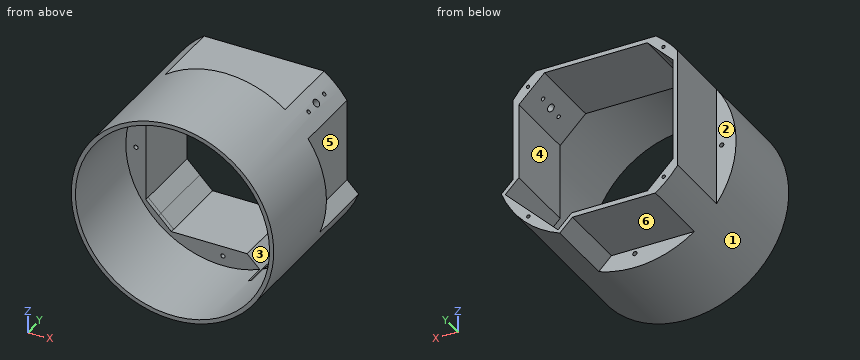
```python
from build123d import *

# Parameters (mm, degrees)
CROQUIS1_R              = 120
CROQUIS1_R_2            = 115
SALIENTE_EXTRUIR1_DEPTH = 110
CROQUIS2_R              = 120
CROQUIS2_W              = 152.253442708
CROQUIS2_H              = 152.577386202
SALIENTE_EXTRUIR2_DEPTH = 90
CORTAR_EXTRUIR1_START   = -85
CORTAR_EXTRUIR1_DEPTH   = 85
CORTAR_EXTRUIR2_DEPTH   = 30
CROQUIS5_R              = 2
CORTAR_EXTRUIR3_DEPTH   = 10
CROQUIS7_R              = 4.5
CORTAR_EXTRUIR4_DEPTH   = 343.045214483
CROQUIS8_R              = 2.25
CORTAR_EXTRUIR5_DEPTH   = 30
CROQUIS12_R             = 2.5
CORTAR_EXTRUIR7_DEPTH   = 15


with BuildPart() as part:
    # Croquis1 → Saliente-Extruir1 (new body)
    with BuildSketch(Plane(origin=(0, 0, 0), x_dir=(1, 0, 0), z_dir=(0, 1, 0))):
        with Locations(Location((0, 0, 0), (0, 0, 270))):
            Circle(CROQUIS1_R)
        with Locations(Location((0, 0, 0), (0, 0, 270))):
            Circle(CROQUIS1_R_2, mode=Mode.SUBTRACT)
    extrude(amount=SALIENTE_EXTRUIR1_DEPTH)

    # Croquis2 → Saliente-Extruir2 (add)
    with BuildSketch(Plane(origin=(0, 110, 0), x_dir=(1, 0, 0), z_dir=(0, 1, 0))):
        with Locations(Location((0, 0, 0), (0, 0, 270))):
            Circle(CROQUIS2_R)
        Rectangle(CROQUIS2_W, CROQUIS2_H, mode=Mode.SUBTRACT)
    extrude(amount=SALIENTE_EXTRUIR2_DEPTH)

    # Croquis3 → Cortar-Extruir1 (cut)
    with BuildSketch(Plane(origin=(0, 200, 0), x_dir=(1, 0, 0), z_dir=(0, 1, 0)).offset(CORTAR_EXTRUIR1_START)):
        Polygon((-45.841188947, 76.288693101), (43.949902098, 76.288693101), (28.807150506, 91.431444693), (-61.004991492, 91.431444693), align=None)
        Polygon((-91.267423391, -61.169009949), (-76.126721354, -46.007259807), (-76.126721354, 45.961058747), (-91.267423391, 61.101790004), align=None)
        Polygon((-61.028027907, -91.408376254), (61.007038201, -91.408376254), (45.887355048, -76.288693101), (-45.887325869, -76.288693101), align=None)
        Polygon((76.126721354, -46.007289027), (91.267423391, -61.147991064), (91.267423391, 28.971171808), (76.126721354, 44.111873845), align=None)
        with BuildLine():
            Line((98.300064852, 29.330876538), (98.300064852, -68.82657372))
            ThreePointArc((98.300064852, -68.82657372), (114.446511048, -36.083183186), (120, 0))
            ThreePointArc((120, 0), (119.08657738, 14.777925699), (116.360215201, 29.330876538))
            Line((116.360215201, 29.330876538), (98.300064852, 29.330876538))
        make_face()
        with BuildLine():
            Line((71.118639022, -96.654742169), (-71.118639022, -96.654742169))
            ThreePointArc((-71.118639022, -96.654742169), (0, -120), (71.118639022, -96.654742169))
        make_face()
        with BuildLine():
            Line((-96.908612184, -70.772317219), (-96.908612184, 70.772317219))
            ThreePointArc((-96.908612184, 70.772317219), (-120, 0), (-96.908612184, -70.772317219))
        make_face()
        with BuildLine():
            ThreePointArc((27.732572497, 116.751464328), (-23.555261835, 117.665413949), (-70.538900009, 97.078646393))
            Line((-70.538900009, 97.078646393), (27.732572497, 97.078646393))
            Line((27.732572497, 97.078646393), (27.732572497, 116.751464328))
        make_face()
        Polygon((76.126721354, 44.111873845), (91.267423391, 28.971171808), (107.376851904, 45.080600321), (91.267423391, 61.190028833), (61.007038201, 91.408376254), (44.895560134, 107.519854321), (28.807150506, 91.431444693), (43.949902098, 76.288693101), (76.126721354, 76.288693101), align=None)
        Polygon((61.007038201, -91.408376254), (76.126721354, -76.288693101), (45.887355048, -76.288693101), align=None)
        Polygon((76.126721354, -46.007289027), (76.126721354, -76.288693101), (91.267423391, -61.147991064), align=None)
        Polygon((-91.267423391, -61.169009949), (-76.126721354, -76.288693101), (-76.126721354, -46.007259807), align=None)
        Polygon((-76.126721354, -76.288693101), (-61.028027907, -91.408376254), (-45.887325869, -76.288693101), align=None)
        Polygon((-91.267423391, 61.101790004), (-76.126721354, 45.961058747), (-76.126721354, 76.288693101), align=None)
        Polygon((-76.126721354, 76.288693101), (-45.841188947, 76.288693101), (-61.004991492, 91.431444693), align=None)
        with BuildLine():
            Line((27.732572497, 116.751464328), (27.732572497, 97.078646393))
            Line((27.732572497, 97.078646393), (42.772301896, 112.118375793))
            ThreePointArc((42.772301896, 112.118375793), (35.32846877, 114.68173043), (27.732572497, 116.751464328))
        make_face()
        with BuildLine():
            ThreePointArc((116.360215201, 29.330876538), (114.392817368, 36.253045866), (112.014025768, 43.044837453))
            Line((112.014025768, 43.044837453), (98.300064852, 29.330876538))
            Line((98.300064852, 29.330876538), (116.360215201, 29.330876538))
        make_face()
    extrude(amount=CORTAR_EXTRUIR1_DEPTH, mode=Mode.SUBTRACT)

    # Croquis4 → Cortar-Extruir2 (cut)
    with BuildSketch(Plane(origin=(0, 115, 0), x_dir=(1, 0, 0), z_dir=(0, 1, 0))):
        Polygon((-91.267423391, 61.101790004), (-91.267423391, -61.169009949), (-61.028027907, -91.408376254), (61.007038201, -91.408376254), (91.267423391, -61.147991064), (91.267423391, 28.971171808), (107.376851904, 45.080600321), (44.895560134, 107.519854321), (28.807150506, 91.431444693), (-61.004991492, 91.431444693), align=None)
    extrude(amount=-CORTAR_EXTRUIR2_DEPTH, mode=Mode.SUBTRACT)

    # Croquis5 → Cortar-Extruir3 (cut)
    with BuildSketch(Plane(origin=(0, 200, 0), x_dir=(1, 0, 0), z_dir=(0, 1, 0))):
        with Locations(Location((80.009543849, 80.403081156, 0), (0, 0, 270))):
            Circle(CROQUIS5_R)
        with Locations(Location((-80.403081156, 80.009543849, 0), (0, 0, 270))):
            Circle(CROQUIS5_R)
        with Locations(Location((-80.009543849, -80.403081156, 0), (0, 0, 270))):
            Circle(CROQUIS5_R)
        with Locations(Location((80.403081156, -80.009543849, 0), (0, 0, 270))):
            Circle(CROQUIS5_R)
    extrude(amount=-CORTAR_EXTRUIR3_DEPTH, mode=Mode.SUBTRACT)

    # Croquis7 → Cortar-Extruir4 (cut, through all)
    with BuildSketch(Plane(origin=(76.207707227, 0, 76.207707227), x_dir=(-0.7071067811865415, 0, 0.7071067811865537), z_dir=(-0.7071067811865537, 0, -0.7071067811865415))):
        with Locations((0, 157.851936769)):
            Circle(CROQUIS7_R)
    extrude(amount=-CORTAR_EXTRUIR4_DEPTH, mode=Mode.SUBTRACT)

    # Croquis8 → Cortar-Extruir5 (cut)
    with BuildSketch(Plane(origin=(76.207707227, 0, 76.207707227), x_dir=(-0.7071067811865415, 0, 0.7071067811865537), z_dir=(-0.7071067811865537, 0, -0.7071067811865415))):
        with Locations((1.055799094, 176.265297527)):
            Circle(CROQUIS8_R)
        with Locations((-0.790662854, 139.817237098)):
            Circle(CROQUIS8_R)
    extrude(amount=-CORTAR_EXTRUIR5_DEPTH, mode=Mode.SUBTRACT)

    # Croquis12 → Cortar-Extruir7 (cut)
    with BuildSketch(Plane(origin=(0, 115, 0), x_dir=(1, 0, 0), z_dir=(0, 1, 0))):
        with Locations(Location((102.928666222, 0, 0), (0, 0, 270))):
            Circle(CROQUIS12_R)
        with Locations(Location((0, -102.928666222, 0), (0, 0, 270))):
            Circle(CROQUIS12_R)
        with Locations(Location((-102.928666222, 0, 0), (0, 0, 270))):
            Circle(CROQUIS12_R)
        with Locations(Location((0, 102.928666222, 0), (0, 0, 270))):
            Circle(CROQUIS12_R)
    extrude(amount=-CORTAR_EXTRUIR7_DEPTH, mode=Mode.SUBTRACT)


solid = part.part
```
The model under review builds one solid part; all positions refer to its coordinate system, in mm. Face numbers are marked on the shaded views. A direction names the side the tool comes from. Coordinates: 2 decimals unless noted, no trailing zeros. Order: outer loops, then holes, each group sorted by start corner. A loop starts at its lowest first (then second) coordinate and runs counter-clockwise, first axis right, second up. Notation, with made-up numbers: (-39, 0.5) -> (9, 0.5) arc R11 ccw to (9, 20.5) -> close; hole circle Ø9 at (10.5, 78). An arc over 180 degrees is marked (long way). Answer in a Markdown table with one row per item. Add a question column.
Item 1: We need section B-B on z = -38.5. Write out the cut boundary in (x, y), plus the area to 3 significant figures.
Item 2: Machinability: for the marked faces 4, 5 and 6, which of the approach directions +Z, -Z, +X, -X, +Y, -Y give a long, thin tool a straight path to every point of the face, cutting with its end or side? Answer none if there is none.
Item 3: We need section D-D on y = 68. Write out the cut boundary in (x, z).
Item 4: Mouldability with a two-part tool opening along Z and no side actions: class the marked faces 1, 2 and 3 as +Z half, -Z half, draft (parallel to the pull), parting line (faces both ways), or undercut.
Item 5: We need section A-A on y = 126.5. Write out the cut boundary in (x, z) (3 decimals).
Item 6: To check wall thickness, follow probe 1 along X at (y, z) = (112.8, 0); probe 2 along Z at (x, y) = (-48.5, 177.5); probe 3 along X at (y, z) = (139.5, -29). State the ranges of each line that lie inside material, in increasing order.
Item 7: We need section C-C on x = 22.5. Write out the cut boundary in (y, z), plus the area to 3 significant figures.
Item 8: Clearance check with flat-ended pins moving along their axes: pin 1 (1.5 mm diameter, centred on y = 127.5, z = -87.5, fed in from -X); pin 2 (1 mm diameter, centred on y = 58, z = 50.5, fed in from +X); pin 3 (1.5 mm diameter, centred on x = 76.5, y = 138.5, fed in from +Z). State where each tip first meets the part, or that it passes through.
Final values:
| question | item | result |
|---|---|---|
| 1 | outline | (-113.66, 0) -> (-108.36, 0) -> (-108.36, 110) -> (-91.27, 110) -> (-91.27, 200) -> (-96.91, 200) -> (-96.91, 115) -> (-113.66, 115) -> close; (100.8, 110) -> (108.36, 110) -> (108.36, 0) -> (113.66, 0) -> (113.66, 115) -> (107.47, 115) -> (107.47, 200) -> (100.8, 200) -> close |
| 1 | area | 2,390 mm2 |
| 2 | face 4 | +Y, -Y |
| 2 | face 5 | +Z, +X, +Y |
| 2 | face 6 | -Z, -X, +Y |
| 3 | outline | circle Ø240 at (0, 0); hole circle Ø230 at (0, 0) |
| 4 | face 1 | parting line |
| 4 | face 2 | draft |
| 4 | face 3 | undercut |
| 5 | outline | (-96.909, -70.772) arc R120 ccw to (-70.539, -97.079) -> (27.733, -97.079) -> (42.772, -112.118) arc R120 ccw to (112.014, -43.045) -> (98.3, -29.331) -> (98.3, 68.827) arc R120 ccw to (71.119, 96.655) -> (-71.119, 96.655) arc R120 ccw to (-96.909, 70.772) -> close; hole (-91.267, -61.102) -> (-76.127, -76.289) -> (-61.005, -91.431) -> (28.807, -91.431) -> (44.896, -107.52) -> (61.007, -91.408) -> (91.267, -61.19) -> (107.377, -45.081) -> (91.267, -28.971) -> (91.267, 61.148) -> (61.007, 91.408) -> (-61.028, 91.408) -> (-76.127, 76.289) -> (-91.267, 61.169) -> close |
| 6 | probe 1 | x = -120 to -105.43, -100.43 to -91.27, 91.27 to 100.43, 105.43 to 120 |
| 6 | probe 2 | z = -97.08 to -91.43, 91.41 to 96.65 |
| 6 | probe 3 | x = -96.91 to -91.27, 91.3 to 98.3 |
| 7 | outline | (0, -117.87) -> (115, -117.87) -> (115, -97.08) -> (200, -97.08) -> (200, -91.43) -> (110, -91.43) -> (110, -112.78) -> (0, -112.78) -> close; (0, 112.78) -> (110, 112.78) -> (110, 91.41) -> (200, 91.41) -> (200, 96.65) -> (115, 96.65) -> (115, 117.87) -> (0, 117.87) -> close |
| 7 | area | 2,310 mm2 |
| 8 | pin 1 | stops at x = -82.91 |
| 8 | pin 2 | stops at x = 109.09 |
| 8 | pin 3 | stops at z = 93.07 |
